Here's how the part is built. I have some questions about the finished solid (model axes, mm). Face numbers are marked on the shaded views. A direction names the side the tool comes from. Give positions to 0.01 mm unless a question says otherwise; leave off trailing zeros. Write each loop counter-clockwise with the first axis right and the second up, starting at its lowest first coordinate (ties: lowest second). Pieces come first, ordered by that corner, then holes. Notation, with made-up numbers: (-34.5, -14.75) - (-2.5, -14.75) arc R33 ccw to (-2.5, 14.25) - close; hole circle Ø11 at (19.25, -15). An arc over 180 degrees is marked (long way). Use a Markdown table: item, result.
```python
from build123d import *

# Parameters (mm, degrees)
SKETCH1_W          = 50.8
SKETCH1_H          = 28.575
EXTRUDE1_DEPTH     = 46.7868
LPATTERN1_COUNT    = 2
LPATTERN1_PITCH    = 27.94
SKETCH5_R          = 13.5001
EXTRUDE2_DEPTH     = 5.969
SKETCH6_W          = 6.3373
SKETCH6_H          = 10.541
CUT_EXTRUDE4_DEPTH = 30.48
HOLE1_D            = 7.137
HOLE1_DEPTH        = 46.7868
HOLE2_D            = 7.137
HOLE2_DEPTH        = 28.575
EXTRUDE3_DEPTH     = 6.779


with BuildPart() as part:
    # Sketch1 → Extrude1 (new body)
    with BuildSketch(Plane(origin=(0, 0, 0), x_dir=(0, 0, -1), z_dir=(1, 0, 0))):
        with Locations((2.3876, 0)):
            Rectangle(SKETCH1_W, SKETCH1_H)
    extrude(amount=EXTRUDE1_DEPTH)

    # S2D0002 → Cut-Revolve1 (revolve, cut)
    with BuildSketch(Plane(origin=(0, 4.7625, 0), x_dir=(-1, 0, 0), z_dir=(0, 1, 0)), mode=Mode.PRIVATE) as cut_revolve1_sk:
        Polygon((-14.5415, -27.5336), (-18.161, -27.5336), (-18.161, -27.7876), (-9.525, -27.7876), (-9.525, -14.0716), (-13.9446, -14.0716), (-13.9446, -26.9113), (-14.5415, -27.5082), align=None)
    cut_revolve1 = revolve(cut_revolve1_sk.sketch.rotate(Axis((9.525, 4.7625, -19.13842003), (0, 0, 1)), 180), axis=Axis((9.525, 4.7625, -19.13842003), (0, 0, 1)), mode=Mode.SUBTRACT)  # turned: the seam where the file's is

    # LPattern1: Cut-Revolve1 ×2
    with Locations(*[(i * LPATTERN1_PITCH, 0, 0) for i in range(1, LPATTERN1_COUNT)]):
        add(cut_revolve1, mode=Mode.SUBTRACT)

    # Sketch5 → Extrude2 (add)
    with BuildSketch(Plane.ZY):
        Circle(SKETCH5_R)
    extrude(amount=EXTRUDE2_DEPTH)

    # Sketch6 → Revolve1 (revolve)
    with BuildSketch(Plane(origin=(0, 0, 0), x_dir=(0, 0, 1), z_dir=(0, -1, 0)), mode=Mode.PRIVATE) as revolve1_sk:
        with Locations((-3.16865, 11.2395)):
            Rectangle(SKETCH6_W, SKETCH6_H)
    revolve(revolve1_sk.sketch.rotate(Axis((5.754582971, 0, 0), (-1, 0, 0)), 180), axis=Axis((5.754582971, 0, 0), (-1, 0, 0)))  # turned: the seam where the file's is

    # S2D0001 → Cut-Revolve4 (revolve, cut)
    with BuildSketch(Plane(origin=(-18.511260017, 3.2639, 0), x_dir=(0, 1, 0), z_dir=(0, 0, 1)), mode=Mode.PRIVATE) as cut_revolve4_sk:
        Polygon((-0.7493, -3.365076823), (-0.7493, -18.003260017), (-3.2639, -19.51418413), (-3.2639, -2.001260017), (0.0381, -2.001260017), align=None)
    revolve(cut_revolve4_sk.sketch.rotate(Axis((0, 0, 0), (-1, 0, 0)), 90), axis=Axis((0, 0, 0), (-1, 0, 0)), mode=Mode.SUBTRACT)  # turned: the seam where the file's is

    # Sketch8 → Cut-Revolve5 (revolve, cut)
    with BuildSketch(Plane(origin=(0, 0, 0), x_dir=(0, 0, -1), z_dir=(0, 1, 0)), mode=Mode.PRIVATE) as cut_revolve5_sk:
        with BuildLine():
            Line((-6.3373, 10.1854), (-6.096, 10.9474))
            Line((-6.096, 10.9474), (-6.096, 15.494))
            ThreePointArc((-6.096, 15.494), (-5.995678675, 16.037796865), (-5.707922533, 16.51))
            Line((-5.707922533, 16.51), (-6.3373, 16.51))
            Line((-6.3373, 16.51), (-6.3373, 10.1854))
        make_face()
    revolve(cut_revolve5_sk.sketch.rotate(Axis((-12.65936, 0, 0), (-1, 0, 0)), 180), axis=Axis((-12.65936, 0, 0), (-1, 0, 0)), mode=Mode.SUBTRACT)  # turned: the seam where the file's is

    # Sketch12 → Cut-Extrude4 (cut, symmetric)
    with BuildSketch(Plane(origin=(0, 0, 0), x_dir=(0, -1, 0), z_dir=(0, 0, -1))):
        Polygon((5.461, 16.51), (5.461, 11.7348), (6.096, 11.0998), (6.096, 16.51), align=None)
        Polygon((-5.461, 16.51), (-5.461, 11.7348), (-6.096, 11.0998), (-6.096, 16.51), align=None)
    extrude(amount=CUT_EXTRUDE4_DEPTH, both=True, mode=Mode.SUBTRACT)

    # Hole1
    with Locations(Plane.ZY):
        with Locations((-16.6878, -7.9248), (16.6624, 7.9502)):
            Hole(HOLE1_D / 2, depth=HOLE1_DEPTH)

    # Hole2
    with Locations(Plane(origin=(0, 14.2875, 0), x_dir=(-1, 0, 0), z_dir=(0, 1, 0))):
        with Locations((-23.3172, -16.6878), (-23.3172, 16.6624)):
            Hole(HOLE2_D / 2, depth=HOLE2_DEPTH)

    # Sketch18 → Extrude3 (add)
    with BuildSketch(Plane(origin=(0, 0, -27.5336), x_dir=(-1, 0, 0), z_dir=(0, 0, -1))):
        Polygon((-2.54, 8.79529163), (-9.525, 12.828083261), (-16.51, 8.79529163), (-16.51, 0.72970837), (-9.525, -3.303083261), (-2.54, 0.72970837), align=None)
    extrude(amount=EXTRUDE3_DEPTH)

    # Sketch19 → Cut-Revolve6 (revolve, cut)
    with BuildSketch(Plane(origin=(0, 4.7625, 0), x_dir=(-1, 0, 0), z_dir=(0, 1, 0)), mode=Mode.PRIVATE) as cut_revolve6_sk:
        with BuildLine():
            Line((-15.748, -34.3126), (-15.748, -36.7256))
            Line((-15.748, -36.7256), (-18.923, -36.7256))
            Line((-18.923, -36.7256), (-18.923, -33.5506))
            Line((-18.923, -33.5506), (-16.51, -33.5506))
            ThreePointArc((-16.51, -33.5506), (-16.286815367, -34.089415367), (-15.748, -34.3126))
        make_face()
    revolve(cut_revolve6_sk.sketch.rotate(Axis((9.525, 4.7625, -18.51025594), (0, 0, -1)), 180), axis=Axis((9.525, 4.7625, -18.51025594), (0, 0, -1)), mode=Mode.SUBTRACT)  # turned: the seam where the file's is


solid = part.part
```
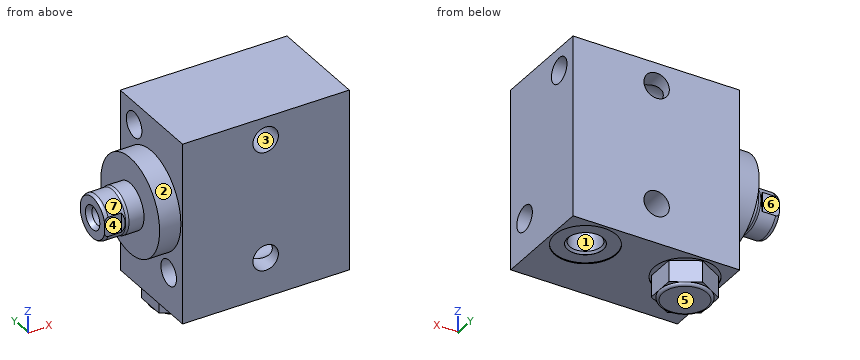
Item 1: If we section it at A-A, the plane y = -10: Write out the boundary of the cut face in (x, z), plus the area to 3 significant figures.
Values:
| item | result |
|---|---|
| outline | (-5.97, -9.07) - (0, -9.07) - (0, -13.78) - (21.24, -13.78) arc R3.57 cw to (25.39, -13.78) - (46.79, -13.78) - (46.79, 23.01) - (0, 23.01) - (0, 9.07) - (-5.97, 9.07) - close; (0, -27.79) - (46.79, -27.79) - (46.79, -19.59) - (25.39, -19.59) arc R3.57 cw to (21.24, -19.59) - (0, -19.59) - close; hole circle Ø7.14 at (23.32, 16.66) |
| area | 2,170 mm2 |
Item 2: If we section it at D-D, the plane z = -8.5: Write out the boundary of the cut face in (x, y).
Values:
| item | result |
|---|---|
| outline | (-5.97, -10.49) - (0, -10.49) - (0, -14.29) - (46.79, -14.29) - (46.79, 14.29) - (0, 14.29) - (0, 10.49) - (-5.97, 10.49) - close |
Item 3: Thinking about a two-plate mould opening in Y: for the marked faces 1, 2 and 3, which applies, +Y half, -Y half, draft (parallel to the pull), parting line (faces both ways), or undercut?
Values:
| item | result |
|---|---|
| face 1 | undercut |
| face 2 | parting line |
| face 3 | draft |
Item 4: For the marked faces 4, 5, 6 and 7, which set-ups out of +Z, -Z, +X, -X, +Y, -Y let a thin tool reach every point of the face, with its end or its side?
Values:
| item | result |
|---|---|
| face 4 | +Z, -Z, -X, -Y |
| face 5 | -Z, +X, -X, +Y, -Y |
| face 6 | +Z, -Z, -X, +Y |
| face 7 | -X |
Item 5: Will these pins go through, and if not, where does the flat tip stop? pin 1 Ø4 at (x, y) = (12.5, -10.5) entering from -Z; pin 2 Ø8 at (y, z) = (-3.5, -21) entering from -X; pin 3 Ø6 at (x, y) = (-4, 10.5) entering from -Z.
Values:
| item | result |
|---|---|
| pin 1 | stops at z = -27.79 |
| pin 2 | stops at x = 0 |
| pin 3 | stops at z = -11.23 |
Item 6: I need wall thicknesses on line 1 along Z through (x, y) = (20.5, 0.25); line 2 along X through (y, z) = (3, -27); line 3 along Z through (x, y) = (24, -4). Which ranges of each line are inside material? Lowest first, please. Write a range as [from, to].
Values:
| item | result |
|---|---|
| line 1 | z = [-27.79, -18.88], [-14.5, 14.47], [18.85, 23.01] |
| line 2 | x = [0, 5.38], [13.67, 33.32], [41.61, 46.79] |
| line 3 | z = [-27.79, -20.19], [-13.19, 13.16], [20.16, 23.01] |
Item 7: If we section it at C-C, the plane x = 31: Write out the boundary of the cut face in (y, z), plus the area to 3 significant figures.
Values:
| item | result |
|---|---|
| outline | (-14.29, -27.79) - (-0.96, -27.79) - (-0.96, -27.53) - (10.49, -27.53) - (10.49, -27.79) - (14.29, -27.79) - (14.29, 23.01) - (-14.29, 23.01) - close; hole circle Ø7.14 at (-7.92, -16.69); hole circle Ø7.14 at (7.95, 16.66) |
| area | 1,370 mm2 |
Item 8: If we section it at B-B, the plane z = 9: Write out the boundary of the cut face in (x, y).
Values:
| item | result |
|---|---|
| outline | (-5.97, -10.06) - (0, -10.06) - (0, -14.29) - (46.79, -14.29) - (46.79, 14.29) - (0, 14.29) - (0, 10.06) - (-5.97, 10.06) - close |
